Geometry: final body of the model. Coordinates: model frame, mm. A direction names the side the tool comes from. Coordinates: 2 decimals unless noted, no trailing zeros. Loops run counter-clockwise (first coordinate to the right, second up) from the corner with the lowest first, then second, coordinate; pieces in that order, holes last. Notation, with made-up numbers: M -16,-24.75 L 26,-24.75 A13 ccw 26,-20.75 Z; hole C 21.25,75.25 d3. An arc over 180 degrees is marked long. Write item = value, one per line. Start each with the question number.
```python
from build123d import *

# Parameters (mm, degrees)
IZIM1_R                     = 14
Y_KSEKLIK_EKSTR_ZYON1_DEPTH = 5.6
Y_KSEKLIK_EKSTR_ZYON2_DEPTH = 5
IZIM3_OUTSIDE_W             = 40.324
IZIM3_OUTSIDE_H             = 49.924
IZIM3_OUTSIDE_R             = 14
KES_EKSTR_ZYON1_DEPTH       = 6.6
KES_EKSTR_ZYON2_DEPTH       = 10
IZIM5_R                     = 2.5
KES_EKSTR_ZYON3_DEPTH       = 22.6
IZIM6_W                     = 3.5
IZIM6_H                     = 8
Y_KSEKLIK_EKSTR_ZYON3_DEPTH = 0.1


with BuildPart() as part:
    # Çizim1 → Yükseklik-Ekstrüzyon1 (new body)
    with BuildSketch(Plane(origin=(0, 0, 0), x_dir=(1, 0, 0), z_dir=(0, 1, 0))):
        Circle(IZIM1_R)
    extrude(amount=-Y_KSEKLIK_EKSTR_ZYON1_DEPTH)

    # Çizim2 → Yükseklik-Ekstrüzyon2 (add, symmetric)
    with BuildSketch(Plane(origin=(0, 0, 0), x_dir=(0, 0, -1), z_dir=(1, 0, 0))):
        Polygon((-14, 0), (-14, 1), (-23.6, 1), (-23.6, 16), (5.4, 16), (14, 1), (14, 0), align=None)
    extrude(amount=Y_KSEKLIK_EKSTR_ZYON2_DEPTH, both=True)

    # Çizim3 outside → Kes-Ekstrüzyon1 (cut)
    with BuildSketch(Plane.XZ.offset(5.6)):
        with Locations((0, 4.8)):
            Rectangle(IZIM3_OUTSIDE_W, IZIM3_OUTSIDE_H)
        Circle(IZIM3_OUTSIDE_R, mode=Mode.SUBTRACT)
    extrude(amount=-KES_EKSTR_ZYON1_DEPTH, mode=Mode.SUBTRACT)

    # Çizim4 → Kes-Ekstrüzyon2 (cut)
    with BuildSketch(Plane.XZ.offset(5.6)):
        with BuildLine():
            ThreePointArc((5, -13.076697), (2.542267, -13.767239), (0, -14))
            Line((0, -14), (5, -14))
            Line((5, -14), (5, -13.076697))
        make_face()
        with BuildLine():
            Line((-5, -13.076697), (-5, -14))
            Line((-5, -14), (0, -14))
            ThreePointArc((0, -14), (-2.542267, -13.767239), (-5, -13.076697))
        make_face()
    extrude(amount=-KES_EKSTR_ZYON2_DEPTH, mode=Mode.SUBTRACT)

    # Çizim5 → Kes-Ekstrüzyon3 (cut, through all)
    with BuildSketch(Plane.XZ.offset(5.6)):
        Circle(IZIM5_R)
    extrude(amount=-KES_EKSTR_ZYON3_DEPTH, mode=Mode.SUBTRACT)

    # Çizim6 → Yükseklik-Ekstrüzyon3 (add)
    with BuildSketch(Plane(origin=(0, 6.288333, -10.968022), x_dir=(-1, 0, 0), z_dir=(0, 0.497384, -0.86753))):
        with Locations((0, 1.932636)):
            Rectangle(IZIM6_W, IZIM6_H)
    extrude(amount=Y_KSEKLIK_EKSTR_ZYON3_DEPTH)


solid = part.part
```
Item 1: Reachability of faces 4 (the flat face through (0, 8, 23.6)), 5 (the cylindrical face through (-13.986, -2.346, 0.616)), 6 (the flat face through (-5, 8, 5)), 7 (the flat face through (8, 0, 0)) from +Z, -Z, +X, -X, +Y, -Y: full face, straight path, thin tool, end or side. Return the list, or none.
Item 2: Pull-direction query (X, two-part tool) for faces 1 (the flat face through (5, 8, 5)), 2 (the flat face through (0, 16, 9)), 3 (the cylindrical face through (-0.54, 5.05, -2.44)); classes: released by +X, released by -X, zero draft, split by the parting line, or undercut.
Item 3: Section query C-C (y = -3). Return the cut outline in (x, z).
Item 4: Section query D-D (y = 7). Return the cut outline in (x, z).
Item 5: Section query B-B (x = 0.75). Return the cut outline in (y, z), plus the area to 3 significant figures.
Item 6: Section query A-A (z = 0). Return the cut outline in (x, y), plus the area to 3 significant figures.
Item 7: First-contact query: pin 1 (5 mm diameter, centred on x = -0.5, z = 21, fed in from -Y); pin 2 (10 mm diameter, centred on y = 6, z = -9, fed in from +X); pin 3 (1.5 mm diameter, centred on y = 2.5, z = 3.5, fed in from -X); pin 4 (3 mm diameter, centred on x = 0, z = 0, fed in from -Y). Flat tips, straight axial feed; report the tip coordinate or a pass-through.
Item 8: Line query: line 1 (X direction, y = 15, z = 4.5); line 2 (Y direction, x = -1.25, z = 14.5); line 3 (X direction, y = -1.5, z = 0.5). Output: solid intervals per line, ascending. Write a range as from..to.
Verdict:
q1.face_4 = +Z, +X, -X, +Y, -Y
q1.face_5 = -Y
q1.face_6 = +Z, -Z, -X, +Y
q1.face_7 = +Z, -Z, +X, +Y
q2.face_1 = released by +X
q2.face_2 = zero draft
q2.face_3 = undercut
q3.outline = C 0,0 d28; hole C 0,0 d5
q4.outline = M -5,-10.56 L -1.75,-10.56 L -1.75,-10.68 L 1.75,-10.68 L 1.75,-10.56 L 5,-10.56 L 5,23.6 L -5,23.6 Z; hole C 0,0 d5
q5.outline = M -5.6,-13.98 L 1.04,-13.98 L 4.49,-12 L 4.54,-12.08 L 11.48,-8.1 L 11.44,-8.02 L 16,-5.4 L 16,-2.38 L -5.6,-2.38 Z; M -5.6,2.38 L 16,2.38 L 16,23.6 L 1,23.6 L 1,13.98 L -5.6,13.98 Z
q5.area = 582 mm2
q6.outline = M -14,-5.6 L -2.5,-5.6 L -2.5,16 L -5,16 L -5,0 L -14,0 Z; M 2.5,-5.6 L 14,-5.6 L 14,0 L 5,0 L 5,16 L 2.5,16 Z
q6.area = 209 mm2
q7.pin_1 = 1
q7.pin_2 = 5
q7.pin_3 = -5
q7.pin_4 = through
q8.line_1 = -5..5
q8.line_2 = 1..16
q8.line_3 = -13.99..-2.45, 2.45..13.99
